The listing builds one solid part. Answer for the finished solid, in the listing's coordinates (mm). Face numbers are marked on the shaded views. A direction names the side the tool comes from. Round coordinates to 2 decimals unless told otherwise and drop trailing zeros. Order: outer loops, then holes, each group sorted by start corner. A loop starts at its lowest first (then second) coordinate and runs counter-clockwise, first axis right, second up. Notation, with made-up numbers: (68, -25.5) -> (111, -25.5) arc R20 ccw to (111, 9.5) -> close; hole circle Ø6 at (47.25, 81.5). An arc over 180 degrees is marked (long way). Return JSON: item names as keys, results as strings. Group by question number.
(1) Each of these flat-tipped pins is pushed along its axis until it touches: pin 1 (0.6 mm diameter, centred on x = 0, z = 4, fed in from -Y); pin 2 (4 mm diameter, centred on y = -14, z = 13, fed in from +X); pin 3 (6 mm diameter, centred on x = 6.5, z = 13, fed in from +Y). Where does it stop, or does it pass through?
(2) Consider line 1 (Y direction, x = 6, z = 9.75); line 2 (Z direction, x = 5, y = -14.5); line 3 (X direction, y = -14.5, z = 5.25). Determine where each line is inside the solid, lowest interval first. Write a range as [from, to].
(3) The part is cut by section B-B (y = -11.25). Determine the outline of the cut face in (x, z), plus the area to 3 significant figures.
(4) The part is cut by section C-C (z = 3.5). Determine the outline of the cut face in (x, y).
(5) Determine the mould class of the marked faces 1, 2 and 3 for opening direction Y: +Y half, -Y half, draft (parallel to the pull), parting line (faces both ways), or undercut.
(6) Which of the six approach directions +Z, -Z, +X, -X, +Y, -Y give full straight-line access (tool end or side, diameter ignored) to the marked faces 4, 5, 6, 7 and 8?
(7) The part is cut by section A-A (x = 0). Determine the outline of the cut face in (y, z).
from build123d import *

# Parameters (mm, degrees)
SKETCH1_W           = 45
SKETCH1_H           = 37.5
BOSS_EXTRUDE1_DEPTH = 2
SKETCH2_W           = 40
SKETCH2_H           = 13
BOSS_EXTRUDE2_DEPTH = 7
BOSS_EXTRUDE3_DEPTH = 7
FILLET1_R           = 1
CUT_EXTRUDE1_DEPTH  = 1
SKETCH5_W           = 41
SKETCH5_H           = 14
CUT_EXTRUDE2_DEPTH  = 7
SKETCH6_W           = 11
SKETCH6_H           = 20
BOSS_EXTRUDE5_DEPTH = 12
SKETCH7_W           = 9
SKETCH7_H           = 9
CUT_EXTRUDE3_DEPTH  = 12
SKETCH8_W           = 132.830335996
SKETCH8_H           = 96.675499104
CUT_EXTRUDE4_DEPTH  = 20


with BuildPart() as part:
    # Sketch1 → Boss-Extrude1 (new body)
    with BuildSketch(Plane.XY):
        Rectangle(SKETCH1_W, SKETCH1_H)
    extrude(amount=BOSS_EXTRUDE1_DEPTH)

    # Sketch2 → Boss-Extrude2 (add)
    with BuildSketch(Plane.XY.offset(2)):
        with Locations((0, -11.25)):
            Rectangle(SKETCH2_W, SKETCH2_H)
    extrude(amount=BOSS_EXTRUDE2_DEPTH)

    # Sketch3 → Boss-Extrude3 (add)
    with BuildSketch(Plane.XY.offset(9)):
        Polygon((-1, -7.75), (-1, -6.75), (-15, -6.75), (-15, -15.75), (-1, -15.75), (-1, -14.75), (1, -14.75), (1, -15.75), (15, -15.75), (15, -6.75), (1, -6.75), (1, -7.75), align=None)
    extrude(amount=BOSS_EXTRUDE3_DEPTH)

    # Fillet1
    fillet1_edges = [part.edges().sort_by_distance(p)[0] for p in [
        (-15, -15.75, 12.5),
        (-1, -15.75, 12.5),
        (1, -15.75, 12.5),
        (-15, -6.75, 12.5),
        (15, -15.75, 12.5),
        (15, -6.75, 12.5),
        (1, -6.75, 12.5),
        (-1, -6.75, 12.5),
    ]]
    fillet(fillet1_edges, radius=FILLET1_R - 0.0001)  # a hair under: the kernel refuses the full size

    # Sketch4 → Cut-Extrude1 (cut)
    with BuildSketch(Plane.XY.offset(16)):
        with BuildLine():
            Line((-1.5, -14.75), (-1.5, -7.75))
            ThreePointArc((-1.5, -7.75), (-1.646446609, -7.396446609), (-2, -7.25))
            Line((-2, -7.25), (-14, -7.25))
            ThreePointArc((-14, -7.25), (-14.353553391, -7.396446609), (-14.5, -7.75))
            Line((-14.5, -7.75), (-14.5, -14.75))
            ThreePointArc((-14.5, -14.75), (-14.353553391, -15.103553391), (-14, -15.25))
            Line((-14, -15.25), (-2, -15.25))
            ThreePointArc((-2, -15.25), (-1.646446609, -15.103553391), (-1.5, -14.75))
        make_face()
        with BuildLine():
            Line((1.5, -7.75), (1.5, -14.75))
            ThreePointArc((1.5, -14.75), (1.646446609, -15.103553391), (2, -15.25))
            Line((2, -15.25), (14, -15.25))
            ThreePointArc((14, -15.25), (14.353553391, -15.103553391), (14.5, -14.75))
            Line((14.5, -14.75), (14.5, -7.75))
            ThreePointArc((14.5, -7.75), (14.353553391, -7.396446609), (14, -7.25))
            Line((14, -7.25), (2, -7.25))
            ThreePointArc((2, -7.25), (1.646446609, -7.396446609), (1.5, -7.75))
        make_face()
    extrude(amount=-CUT_EXTRUDE1_DEPTH, mode=Mode.SUBTRACT)

    # Sketch5 → Cut-Extrude2 (cut)
    with BuildSketch(Plane.XY.offset(9)):
        with Locations((0, -11.25)):
            Rectangle(SKETCH5_W, SKETCH5_H)
        with BuildLine():
            Line((-17.5, -8.75), (-15.5, -8.75))
            Line((-15.5, -8.75), (-15.5, -7.75))
            ThreePointArc((-15.5, -7.75), (-15.060660172, -6.689339828), (-14, -6.25))
            Line((-14, -6.25), (-2, -6.25))
            ThreePointArc((-2, -6.25), (-1.133974596, -6.525255129), (-0.585786438, -7.25))
            Line((-0.585786438, -7.25), (0.585786438, -7.25))
            ThreePointArc((0.585786438, -7.25), (1.133974596, -6.525255129), (2, -6.25))
            Line((2, -6.25), (14, -6.25))
            ThreePointArc((14, -6.25), (15.060660172, -6.689339828), (15.5, -7.75))
            Line((15.5, -7.75), (15.5, -8.75))
            Line((15.5, -8.75), (17.5, -8.75))
            ThreePointArc((17.5, -8.75), (20, -11.25), (17.5, -13.75))
            Line((17.5, -13.75), (15.5, -13.75))
            Line((15.5, -13.75), (15.5, -14.75))
            ThreePointArc((15.5, -14.75), (15.060660172, -15.810660172), (14, -16.25))
            Line((14, -16.25), (2, -16.25))
            ThreePointArc((2, -16.25), (1.133974596, -15.974744871), (0.585786438, -15.25))
            Line((0.585786438, -15.25), (-0.585786438, -15.25))
            ThreePointArc((-0.585786438, -15.25), (-1.133974596, -15.974744871), (-2, -16.25))
            Line((-2, -16.25), (-14, -16.25))
            ThreePointArc((-14, -16.25), (-15.060660172, -15.810660172), (-15.5, -14.75))
            Line((-15.5, -14.75), (-15.5, -13.75))
            Line((-15.5, -13.75), (-17.5, -13.75))
            ThreePointArc((-17.5, -13.75), (-20, -11.25), (-17.5, -8.75))
        make_face(mode=Mode.SUBTRACT)
    extrude(amount=-CUT_EXTRUDE2_DEPTH, mode=Mode.SUBTRACT)

    # Sketch6 → Boss-Extrude5 (add)
    with BuildSketch(Plane(origin=(0, 0, 0), x_dir=(-1, 0, 0), z_dir=(0, 0, -1))):
        with Locations((-6, 8.25)):
            Rectangle(SKETCH6_W, SKETCH6_H)
        with Locations((6, 8.25)):
            Rectangle(SKETCH6_W, SKETCH6_H)
    extrude(amount=BOSS_EXTRUDE5_DEPTH)

    # Sketch7 → Cut-Extrude3 (cut)
    with BuildSketch(Plane(origin=(0, 18.25, 0), x_dir=(1, 0, 0), z_dir=(0, 1, 0))):
        with Locations((-6, 5.5)):
            Rectangle(SKETCH7_W, SKETCH7_H)
        with Locations((6, 5.5)):
            Rectangle(SKETCH7_W, SKETCH7_H)
    extrude(amount=-CUT_EXTRUDE3_DEPTH, mode=Mode.SUBTRACT)

    # Sketch8 → Cut-Extrude4 (cut)
    with BuildSketch(Plane.XY.offset(2)):
        Rectangle(SKETCH8_W, SKETCH8_H)
    extrude(amount=-CUT_EXTRUDE4_DEPTH, mode=Mode.SUBTRACT)


solid = part.part
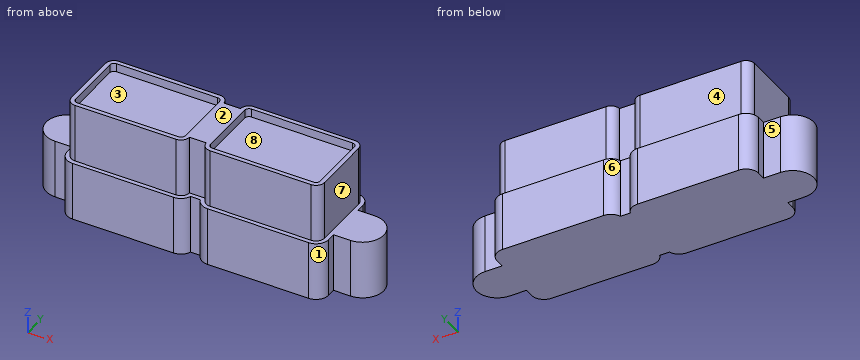
Answer below:
{
 "1": {"pin 1": "stops at y = -15.25", "pin 2": "stops at x = 15", "pin 3": "stops at y = -6.75"},
 "2": {"line 1": "y = [-15.75, -6.75]", "line 2": "z = [2, 15]", "line 3": "x = [-15.5, 15.5]"},
 "3": {"outline": "(-20, 2) -> (20, 2) -> (20, 9) -> (15, 9) -> (15, 16) -> (14.5, 16) -> (14.5, 15) -> (1.5, 15) -> (1.5, 16) -> (-1.5, 16) -> (-1.5, 15) -> (-14.5, 15) -> (-14.5, 16) -> (-15, 16) -> (-15, 9) -> (-20, 9) -> close", "area": "464 mm²"},
 "4": {"outline": "(-17.5, -13.75) -> (-15.5, -13.75) -> (-15.5, -14.75) arc R1.5 ccw to (-14, -16.25) -> (-2, -16.25) arc R1.5 ccw to (-0.59, -15.25) -> (0.59, -15.25) arc R1.5 ccw to (2, -16.25) -> (14, -16.25) arc R1.5 ccw to (15.5, -14.75) -> (15.5, -13.75) -> (17.5, -13.75) arc R2.5 ccw to (17.5, -8.75) -> (15.5, -8.75) -> (15.5, -7.75) arc R1.5 ccw to (14, -6.25) -> (2, -6.25) arc R1.5 ccw to (0.59, -7.25) -> (-0.59, -7.25) arc R1.5 ccw to (-2, -6.25) -> (-14, -6.25) arc R1.5 ccw to (-15.5, -7.75) -> (-15.5, -8.75) -> (-17.5, -8.75) arc R2.5 ccw to start"},
 "5": {"face 1": "-Y half", "face 2": "draft", "face 3": "undercut"},
 "6": {"face 4": "+Z, +X, -X, +Y", "face 5": "+Z, -Z, -X, +Y", "face 6": "+Z, -Z, +Y", "face 7": "+Z, +X, +Y, -Y", "face 8": "+Z"},
 "7": {"outline": "(-15.25, 2) -> (-7.25, 2) -> (-7.25, 9) -> (-7.75, 9) -> (-7.75, 16) -> (-14.75, 16) -> (-14.75, 9) -> (-15.25, 9) -> close"}
}
